CAD build for the part. Positions are in the model's coordinates, mm. A direction names the side the tool comes from. Coordinates: 2 decimals unless noted, no trailing zeros. Loops run counter-clockwise (first coordinate to the right, second up) from the corner with the lowest first, then second, coordinate; pieces in that order, holes last. Notation, with made-up numbers: (19, 83) -> (61, 83) arc R37 ccw to (61, 120) -> close; hole circle Ø5 at (-26, 13). An arc over 180 degrees is marked (long way). Return JSON: item names as keys, results as strings. Group by question number.
(1) Probe L1, parallel to X at y = 2.25, z = 12.5; L2, parallel to X at y = 7, z = 20.5; L3, parallel to X at y = 6.5, z = 8.75. List the from-to ranges inside material, lowest first.
(2) Saw through at A-A on z = 12.7. Write the cut outline in (x, y) (3 decimals), then the cut area to 3 significant figures.
(3) Saw through at C-C on z = 21. Write the cut outline in (x, y) (3 decimals).
(4) Tool access for faces 4 (the face through (-26, 6.35, 13)), 5 (the face through (35.2, 6.35, 12.5)), 6 (the face through (-25, 0, 13)): list every direction of +Z, -Z, +X, -X, +Y, -Y with a clear straight run to the whole face (end or side of a thin tool).
(5) Flat gauge pins, fed straight in: pin 1 Ø12 at (y, z) = (18.5, 4) entering from +X; pin 2 Ø1 at (y, z) = (14, 3) entering from +X; pin 3 Ø1 at (y, z) = (16.5, 14) entering from +X. Where does each tip first touch, or does it go through?
(6) Saw through at D-D on x = 0. Write the cut outline in (y, z) (3 decimals).
(7) Saw through at B-B on y = 3.75. Write the cut outline in (x, z), then the cut area to 3 significant figures.
(8) Mould opens along Z. For faces 1 (the face through (33.89, 3.22, 15.53)), 2 (the face through (-1, 16, 0)), 3 (the face through (-40.4, 3, 13)) say: pulls with the +Z half, pulls with the -Z half, needs draft (parallel to the pull), parting line crosses it, or undercut.
```python
from build123d import *

# Parameters (mm, degrees)
BOSS_EXTRUDE1_DEPTH = 25.4
SKETCH2_R           = 4.191
CUT_EXTRUDE1_DEPTH  = 6.35


with BuildPart() as part:
    # Sketch1 → Boss-Extrude1 (new body)
    with BuildSketch(Plane.XY):
        with BuildLine():
            Line((-40.4, 0), (-15, 0))
            ThreePointArc((-15, 0), (0, 15), (15, 0))
            Line((15, 0), (40.4, 0))
            Line((40.4, 0), (40.4, 6.35))
            Line((40.4, 6.35), (21.298547486, 6.35))
            ThreePointArc((21.298547486, 6.35), (0, 22.225), (-21.298547486, 6.35))
            Line((-21.298547486, 6.35), (-40.4, 6.35))
            Line((-40.4, 6.35), (-40.4, 0))
        make_face()
    extrude(amount=BOSS_EXTRUDE1_DEPTH)

    # Sketch2 → Cut-Extrude1 (cut)
    with BuildSketch(Plane(origin=(0, 6.35, 0), x_dir=(1, 0, 0), z_dir=(0, 1, 0))):
        with Locations(Location((-30.798547486, -12.7, 0), (0, 0, 180))):
            Circle(SKETCH2_R)
        with Locations(Location((30.798553886, -12.7, 0), (0, 0, 180))):
            Circle(SKETCH2_R)
    extrude(amount=-CUT_EXTRUDE1_DEPTH, mode=Mode.SUBTRACT)


solid = part.part
```
Geometry results:
{
 "1": {"L1": "-40.4 to -34.98, -26.61 to -14.83, 14.83 to 26.61, 34.98 to 40.4", "L2": "-21.09 to -13.27, 13.27 to 21.09", "L3": "-21.25 to -13.52, 13.52 to 21.25"},
 "2": {"outline": "(-40.4, 0) -> (-34.99, 0) -> (-34.99, 6.35) -> (-40.4, 6.35) -> close; (-26.608, 0) -> (-15, 0) arc R15 cw to (15, 0) -> (26.608, 0) -> (26.608, 6.35) -> (21.299, 6.35) arc R22.225 ccw to (-21.299, 6.35) -> (-26.608, 6.35) -> close; (34.99, 0) -> (40.4, 0) -> (40.4, 6.35) -> (34.99, 6.35) -> close", "area": "551 mm²"},
 "3": {"outline": "(-40.4, 0) -> (-15, 0) arc R15 cw to (15, 0) -> (40.4, 0) -> (40.4, 6.35) -> (21.299, 6.35) arc R22.225 ccw to (-21.299, 6.35) -> (-40.4, 6.35) -> close"},
 "4": {"face 4": "+Z, -Z, -X, +Y", "face 5": "+Z, -Z, +X, +Y", "face 6": "+Z, -Z, +X, -X, -Y"},
 "5": {"pin 1": "x = 18.38", "pin 2": "x = 17.66", "pin 3": "x = 15.43"},
 "6": {"outline": "(15, 0) -> (22.225, 0) -> (22.225, 25.4) -> (15, 25.4) -> close"},
 "7": {"outline": "(-40.4, 0) -> (-14.52, 0) -> (-14.52, 25.4) -> (-40.4, 25.4) -> close; (14.52, 0) -> (40.4, 0) -> (40.4, 25.4) -> (14.52, 25.4) -> close; hole circle Ø8.38 at (-30.8, 12.7); hole circle Ø8.38 at (30.8, 12.7)", "area": "1,200 mm²"},
 "8": {"face 1": "undercut", "face 2": "pulls with the -Z half", "face 3": "needs draft"}
}
